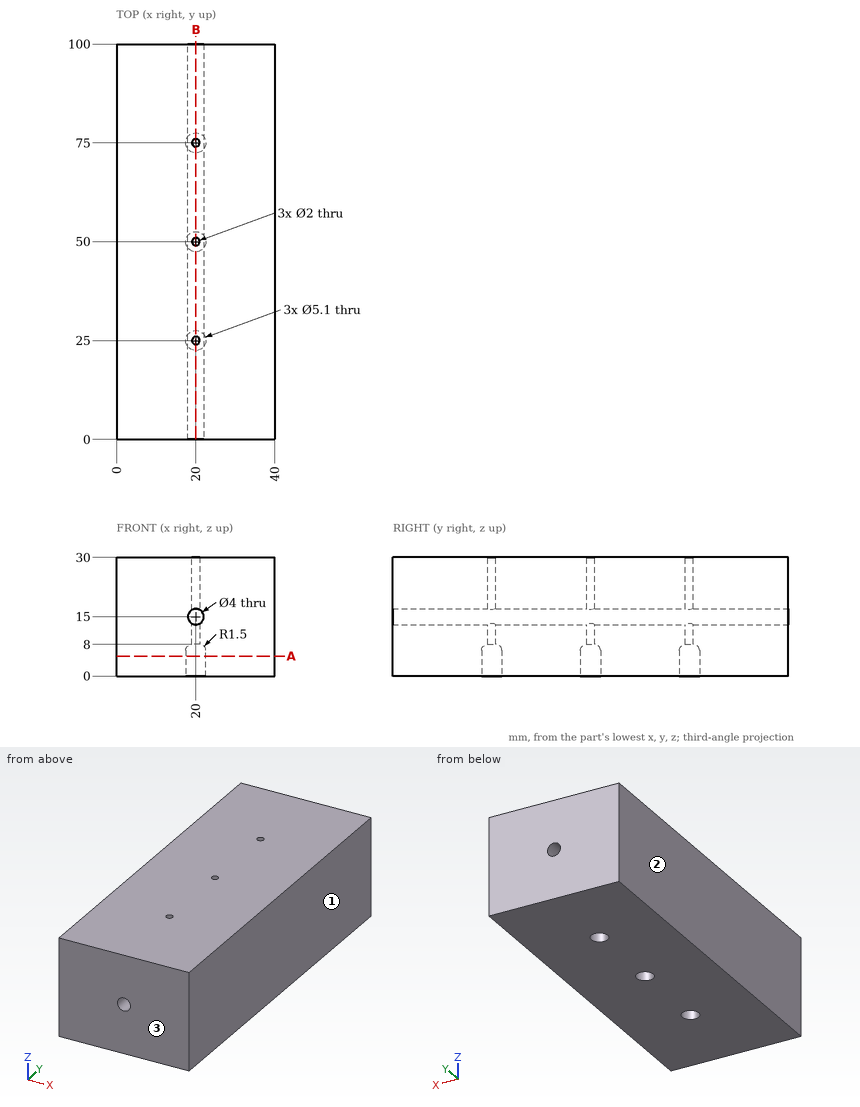
Source: three-view drawing plus pictorial views. Frame: mm from the lowest corner of the part. Give positions to 0.01 mm unless a question says otherwise; leave off trailing zeros. Loops run counter-clockwise (first coordinate to the right, second up) from the corner with the lowest first, then second, coordinate; pieces in that order, holes last.
1) Section query B-B on x = 20. Count the separate pieces of the cut face and the enclosed holes in it, and give its area (3 significant figures).
A:
separate pieces: 8
enclosed holes: 0
area: 2,370 mm2
2) Section query A-A on z = 5. Return the cut outline in (x, y), and give its area (3 significant figures).
A:
outline: (0, 0) - (40, 0) - (40, 100) - (0, 100) - close; hole circle Ø5.1 at (20, 25); hole circle Ø5.1 at (20, 50); hole circle Ø5.1 at (20, 75)
area: 3,940 mm2
3) Line query: L1, parallel to Y at x = 20, z = 9; L2, parallel to Y at x = 20, z = 2; L3, parallel to Z at x = 19.5, y = 11. Output: solid intervals per line, ascending.
A:
L1: y = 0 to 24, 26 to 49, 51 to 74, 76 to 100
L2: y = 0 to 22.45, 27.55 to 47.45, 52.55 to 72.45, 77.55 to 100
L3: z = 0 to 13.06, 16.94 to 30
4) Contact query for flat-ended pins moving along their axis: pin 1 (2.5 mm diameter, centred on x = 20, y = 50, fed in from +Z); pin 2 (3 mm diameter, centred on x = 20, y = 75, fed in from -Z); pin 3 (2.5 mm diameter, centred on x = 20, y = 50, fed in from -Z). Output: stop coordinate, or through.
A:
pin 1: stops at z = 30
pin 2: stops at z = 7.93
pin 3: stops at z = 7.99
5) Mould query, pull axis X, two halves, no side actions, for the marked faces 1, 2 and 3. Classes: released by +X, released by -X, zero draft, split by the parting line, or undercut.
A:
face 1: released by +X
face 2: released by -X
face 3: zero draft
